CAD build for the part. Positions are in the model's coordinates, mm. A direction names the side the tool comes from. Round coordinates to 2 decimals unless told otherwise and drop trailing zeros. Loops run counter-clockwise (first coordinate to the right, second up) from the corner with the lowest first, then second, coordinate; pieces in that order, holes last. Notation, with made-up numbers: M 17,69 L 21,69 A24 cw 21,81 Z; hole C -20.5,1 d4. An arc over 180 degrees is marked long. One line per item, written item: value. Start each with the question number.
from build123d import *

# Parameters (mm, degrees)
F0_W      = 91.5
F0_H      = 61
F1_DEPTH  = 14.5
F2_T      = -1.5
F3_W      = 8
F3_H      = 8
F3_W_2    = 16
F3_H_2    = 7.2
F4_DEPTH  = 2.1
F5_W      = 19.8
F5_H      = 8.7
F6_DEPTH  = 5.8
F7_W      = 16.6
F7_H      = 8.3
F7_W_2    = 15.6
F8_DEPTH  = 3
F9_R      = 3
F9_R_2    = 1.325
F10_DEPTH = 4.7
F11_R     = 0.5


with BuildPart() as f1:
    # F0 (on Top) → F1 (new body)
    with BuildSketch(Plane.XY):
        Rectangle(F0_W, F0_H)
    extrude(amount=F1_DEPTH)

    # F2
    f2_openings = [f1.faces().sort_by_distance(p)[0] for p in [
        (0, 0, 14.5),
    ]]
    offset(amount=F2_T, openings=f2_openings)

    # F3 (on face) → F4 (cut)
    with BuildSketch(Plane.XZ.offset(30.5)):
        with Locations((-32.25, 10.5)):
            Rectangle(F3_W, F3_H)
        with Locations((-11.55, 10.9)):
            Rectangle(F3_W_2, F3_H_2)
        with BuildLine():
            ThreePointArc((6.15, 9.65), (9.3, 6.5), (12.45, 9.65))
            ThreePointArc((12.45, 9.65), (9.3, 12.8), (6.15, 9.65))
        make_face()
        with BuildLine():
            ThreePointArc((6.15, 9.65), (9.3, 12.8), (12.45, 9.65))
            Line((12.45, 9.65), (12.45, 14.5))
            Line((12.45, 14.5), (6.15, 14.5))
            Line((6.15, 14.5), (6.15, 9.65))
        make_face()
    extrude(amount=-F4_DEPTH, mode=Mode.SUBTRACT)

    # F5 (on face) → F6 (cut)
    with BuildSketch(Plane(origin=(-45.75, 0, 0), x_dir=(0, -1, 0), z_dir=(-1, 0, 0))):
        with Locations((-2.006637, 4.35)):
            Rectangle(F5_W, F5_H)
    extrude(amount=-F6_DEPTH, mode=Mode.SUBTRACT)

    # F7 (on face) → F8 (cut)
    with BuildSketch(Plane.YZ.offset(45.75)):
        with Locations((-17.6, 10.35)):
            Rectangle(F7_W, F7_H)
        with Locations((0.5, 10.35)):
            Rectangle(F7_W_2, F7_H)
        with Locations((18.1, 10.35)):
            Rectangle(F7_W_2, F7_H)
    extrude(amount=-F8_DEPTH, mode=Mode.SUBTRACT)

    # F9 (on face) → F10 (join)
    with BuildSketch(Plane.XY.offset(1.5)):
        with Locations((19.04, 24.5)):
            Circle(F9_R)
        with Locations((19.04, 24.5)):
            Circle(F9_R_2, mode=Mode.SUBTRACT)
        with Locations((19.04, -24.5)):
            Circle(F9_R)
        with Locations((19.04, -24.5)):
            Circle(F9_R_2, mode=Mode.SUBTRACT)
        with Locations((-38.96, 24.5)):
            Circle(F9_R)
        with Locations((-38.96, 24.5)):
            Circle(F9_R_2, mode=Mode.SUBTRACT)
        with Locations((-38.96, -24.5)):
            Circle(F9_R)
        with Locations((-38.96, -24.5)):
            Circle(F9_R_2, mode=Mode.SUBTRACT)
    extrude(amount=F10_DEPTH)

    # F11
    f11_edges = [f1.edges().sort_by_distance(p)[0] for p in [
        (-45.75, -30.5, 7.25),
        (-45.75, 30.5, 7.25),
        (45.75, -30.5, 7.25),
        (45.75, 30.5, 7.25),
    ]]
    fillet(f11_edges, radius=F11_R)


solid = f1.part
(1) Probe L1, parallel to Y at x = -38.96, z = 3.65 (3 decimals); L2, parallel to Y at x = -31.5, z = 3; L3, parallel to X at y = 16.5, z = 4.5. List the from-to ranges inside material, lowest first.
(2) Which spindle directions (+Z, -Z, +X, -X, +Y, -Y) get a long thin tool onto all of the face, cutting with end or side? Do faces 5 (the cylindrical face through (16.043, 24.632, 3.817)), 6 (the cylindrical face through (9.2, -29.8, 6.5)), 7 (the flat face through (-45, 11.907, 2)). Say none if no direction does.
(3) Flat gauge pins, fed straight in: P1, Ø2.5, axis at x = 19.04, y = 24.5, coming from the +Z side; P2, Ø1.2, axis at y = 0, z = 0.5, coming from the -X side; P3, Ø3, axis at x = 16.5, y = -21.5, coming from the +Z side. Where does each tip first touch, or does it go through?
(4) Slice it at A-A, the plane z = 3.5. Count the separate pieces of the cut face and the enclosed holes in it, and give its area (3 significant figures).
(5) Slice it at C-C, the plane x = -11. List the corners of the cut face in (y, z).
(6) Mould opens along X. For faces 1 (the flat face through (45.75, 0, 4)), 2 (the flat face through (-1, 0, 0)), 3 (the cylindrical face through (-37.696, -24.102, 3.817)), 4 (the flat face through (-45.75, 0, 9)) say: pulls with the +X half, pulls with the -X half, needs draft (parallel to the pull), parting line crosses it, or undercut.
(7) Slice it at B-B, the plane y = 2. List the corners of the cut face in (x, z).
Check result:
1. L1: y = -30.5 to -29, -27.5 to -25.825, -23.175 to -21.5, 21.5 to 23.175, 25.825 to 27.5, 29 to 30.5
1. L2: y = -30.5 to -29, 29 to 30.5
1. L3: x = -45.75 to -44.25, 44.25 to 45.75
2. face 5: +Z
2. face 6: +Z, -Y
2. face 7: -Z, -X
3. P1: stops at z = 1.5
3. P2: stops at x = -39.95
3. P3: stops at z = 6.2
4. separate pieces: 5
4. enclosed holes: 4
4. area: 510 mm^2
5. outline: M -30.5,0 L 30.5,0 L 30.5,14.5 L 29,14.5 L 29,1.5 L -29,1.5 L -29,7.3 L -30.5,7.3 Z
6. face 1: pulls with the +X half
6. face 2: needs draft
6. face 3: undercut
6. face 4: pulls with the -X half
7. outline: M -45.75,8.7 L -44.25,8.7 L -44.25,14.5 L -45.75,14.5 Z; M -39.95,0 L 45.75,0 L 45.75,6.2 L 44.25,6.2 L 44.25,1.5 L -39.95,1.5 Z
